Input: part model. Units: mm. Frame: model coordinates. A direction names the side the tool comes from. Give positions to 0.01 mm unless a question says otherwise; leave off trailing zeros. Loops run counter-clockwise (first coordinate to the right, second up) from the corner with the lowest first, then second, coordinate; pieces in that order, holes last.
from build123d import *

# Parameters (mm, degrees)
F1_R     = 8
F2_DEPTH = 48
F3_R     = 1.75
F4_DEPTH = 5
F5_R     = 1.75
F6_DEPTH = 50
F7_W     = 4.0019527676
F7_H     = 1
F8_DEPTH = 80


with BuildPart() as f2:
    # F1 (on Right) → F2 (new body)
    with BuildSketch(Plane.YZ):
        with BuildLine():
            ThreePointArc((-11, 14.2537585227), (-10.2225241501, 10.1917393204), (-8, 6.7039240874))
            ThreePointArc((-8, 6.7039240874), (2.1006018341, 3.4561906514), (10.246950766, 10.2537585227))
            ThreePointArc((10.246950766, 10.2537585227), (10.810098483, 12.218624427), (11, 14.2537585227))
            ThreePointArc((11, 14.2537585227), (10.810098483, 16.2888926183), (10.246950766, 18.2537585227))
            ThreePointArc((10.246950766, 18.2537585227), (-2.0351340956, 25.0638570057), (-11, 14.2537585227))
        make_face()
        with Locations((0, 14.2537585227)):
            Circle(F1_R, mode=Mode.SUBTRACT)
        with BuildLine():
            ThreePointArc((-11, -15.2462414773), (-10.2225241501, -11.184222275), (-8, -7.6964070421))
            Line((-8, -7.6964070421), (-8, 6.7039240874))
            ThreePointArc((-8, 6.7039240874), (-10.2225241501, 10.1917393204), (-11, 14.2537585227))
            Line((-11, 14.2537585227), (-11, -15.2462414773))
        make_face()
        with BuildLine():
            ThreePointArc((10.246950766, -19.2462414773), (10.810098483, -17.281375573), (11, -15.2462414773))
            ThreePointArc((11, -15.2462414773), (10.810098483, -13.2111073817), (10.246950766, -11.2462414773))
            ThreePointArc((10.246950766, -11.2462414773), (2.1006018341, -4.4486736061), (-8, -7.6964070421))
            ThreePointArc((-8, -7.6964070421), (-10.2225241501, -11.184222275), (-11, -15.2462414773))
            ThreePointArc((-11, -15.2462414773), (-2.0351340956, -26.0563399604), (10.246950766, -19.2462414773))
        make_face()
        with Locations((0, -15.2462414773)):
            Circle(F1_R, mode=Mode.SUBTRACT)
        with BuildLine():
            ThreePointArc((10.246950766, -11.2462414773), (10.810098483, -13.2111073817), (11, -15.2462414773))
            ThreePointArc((11, -15.2462414773), (10.810098483, -17.281375573), (10.246950766, -19.2462414773))
            Line((10.246950766, -19.2462414773), (16.246950766, -19.2462414773))
            Line((16.246950766, -19.2462414773), (16.246950766, -11.2462414773))
            Line((16.246950766, -11.2462414773), (10.246950766, -11.2462414773))
        make_face()
        with BuildLine():
            ThreePointArc((11, 14.2537585227), (10.810098483, 12.218624427), (10.246950766, 10.2537585227))
            Line((10.246950766, 10.2537585227), (16.246950766, 10.2537585227))
            Line((16.246950766, 10.2537585227), (16.246950766, 18.2537585227))
            Line((16.246950766, 18.2537585227), (10.246950766, 18.2537585227))
            ThreePointArc((10.246950766, 18.2537585227), (10.810098483, 16.2888926183), (11, 14.2537585227))
        make_face()
    extrude(amount=F2_DEPTH)

    # F3 (on face) → F4 (cut)
    with BuildSketch(Plane.XZ.offset(11)):
        with Locations((38.5, 0)):
            Circle(F3_R)
        with Locations((9.5, 0)):
            Circle(F3_R)
    extrude(amount=-F4_DEPTH, mode=Mode.SUBTRACT)

    # F5 (on face) → F6 (cut)
    with BuildSketch(Plane.XY.offset(18.2537585227)):
        with Locations((3.5, 13.246950766)):
            Circle(F5_R)
        with Locations((44.749999574, 13.243720019)):
            Circle(F5_R)
    extrude(amount=-F6_DEPTH, mode=Mode.SUBTRACT)

    # F7 (on face) → F8 (cut)
    with BuildSketch(Plane.YZ.offset(48)):
        with Locations((8.2459743822, 9.7537585227)):
            Rectangle(F7_W, F7_H)
        with Locations((8.2459743822, -10.7462414773)):
            Rectangle(F7_W, F7_H)
    extrude(amount=-F8_DEPTH, mode=Mode.SUBTRACT)


solid = f2.part
(1) Ray query, probe 1 along Z at (x, y) = (11.5, -0.25); probe 2 along Z at (x, y) = (40.5, 15.25); probe 3 along X at (y, z) = (12.5, -16). Return the intervals inside material, ascending.
Values follow:
probe 1: z = -26.24 to -23.24, -7.25 to -4.25, 3.26 to 6.26, 22.25 to 25.25
probe 2: z = -19.25 to -11.25, 10.25 to 18.25
probe 3: x = 0 to 1.92, 5.08 to 43.17, 46.33 to 48
(2) Cut plane B-B (z = 0). Return the cut outline in (x, y), and give its area (3 significant figures).
Values follow:
outline: (0, -11) - (7.75, -11) - (7.75, -8) - (0, -8) - close; (11.25, -11) - (36.75, -11) - (36.75, -8) - (11.25, -8) - close; (40.25, -11) - (48, -11) - (48, -8) - (40.25, -8) - close
area: 123 mm2
(3) Cut plane D-D (y = 0). Return the cut outline in (x, z).
Values follow:
outline: (0, -26.25) - (48, -26.25) - (48, -23.25) - (0, -23.25) - close; (0, -7.25) - (48, -7.25) - (48, -4.25) - (0, -4.25) - close; (0, 3.25) - (48, 3.25) - (48, 6.25) - (0, 6.25) - close; (0, 22.25) - (48, 22.25) - (48, 25.25) - (0, 25.25) - close
(4) Pin query (flat end, axial travel): pin 1 Ø7.5 at (x, y) = (27, 10) entering from -Z; pin 2 Ø6 at (x, y) = (25, -4.5) entering from -Z; pin 3 Ø4 at (x, y) = (44.75, 13.24) entering from -Z; pin 4 Ø9.5 at (y, z) = (0, 14.25) entering from -X. Return the tip coordinate at first contact, or that it passes through.
Values follow:
pin 1: stops at z = -24.3
pin 2: stops at z = -26.14
pin 3: stops at z = -19.25
pin 4: passes through
(5) Cut plane C-C (x = 3.5). Return the cut outline in (y, z) (3 decimals), and give its area (3 significant figures).
Values follow:
outline: (-11, -15.246) arc R11 ccw to (10.247, -19.246) - (11.497, -19.246) - (11.497, -11.246) - (6.928, -11.246) arc R8 cw (long way) to (6.245, -10.246) - (9.798, -10.246) arc R11 ccw to (-8, -7.696) - (-8, 6.704) arc R11 ccw to (9.798, 9.254) - (6.245, 9.254) arc R8 cw (long way) to (6.928, 10.254) - (11.497, 10.254) - (11.497, 18.254) - (10.247, 18.254) arc R11 ccw to (-11, 14.254) - close; (14.997, -19.246) - (16.247, -19.246) - (16.247, -11.246) - (14.997, -11.246) - close; (14.997, 10.254) - (16.247, 10.254) - (16.247, 18.254) - (14.997, 18.254) - close
area: 441 mm2
(6) Reachability of faces 1 (the flat face through (24, 8, 9.254)), 2 (the flat face through (24, 13, -19.246)), 3 (the flat face through (24, 13, 18.254)), 4 (the cylindrical face through (40.117, -9.521, -0.67)) from +Z, -Z, +X, -X, +Y, -Y: full face, straight path, thin tool, end or side. Return the list, or none.
Values follow:
face 1: +X, -X, +Y
face 2: -Z, +X, -X, +Y
face 3: +Z, +X, -X, +Y
face 4: +Y, -Y
(7) Mould query, pull axis Y, two halves, no side actions, for faces 5 (the cylindrical face through (23.664, -2.244, -26.015)), 6 (the cylindrical face through (23.664, -6.406, 19.046)), 7 (the flat face through (24, 16.247, 14)). Classes: +Y half, -Y half, draft (parallel to the pull), parting line (faces both ways), or undercut.
Values follow:
face 5: parting line
face 6: undercut
face 7: +Y half
(8) Cut plane A-A (x = 9.5). Return the cut outline in (y, z) (3 decimals), and give its area (3 significant figures).
Values follow:
outline: (-11, -15.246) arc R11 ccw to (10.247, -19.246) - (16.247, -19.246) - (16.247, -11.246) - (6.928, -11.246) arc R8 cw (long way) to (6.245, -10.246) - (9.798, -10.246) arc R11 ccw to (-8, -7.696) - (-8, -1.75) - (-11, -1.75) - close; (-11, 1.75) - (-8, 1.75) - (-8, 6.704) arc R11 ccw to (9.798, 9.254) - (6.245, 9.254) arc R8 cw (long way) to (6.928, 10.254) - (16.247, 10.254) - (16.247, 18.254) - (10.247, 18.254) arc R11 ccw to (-11, 14.254) - close
area: 486 mm2
